Build history of the part. All positions in model axes, mm. Round coordinates to 2 decimals unless told otherwise and drop trailing zeros. Write each loop counter-clockwise with the first axis right and the second up, starting at its lowest first coordinate (ties: lowest second). Pieces come first, ordered by that corner, then holes. Notation, with made-up numbers: (87, 80.25) -> (123, 80.25) arc R13 cw to (123, 87.25) -> close; hole circle Ø6 at (89, 57). An arc over 180 degrees is marked (long way). One line per question, with ' | ' between items.
Autodesk Inventor part; units mm, degrees
ref_plane "YZ Plane" through (0, 0, 0) normal (1, 0, 0) x (0, 1, 0)
ref_plane "XZ Plane" through (0, 0, 0) normal (0, 1, 0) x (-1, 0, 0)
ref_plane "XY Plane" through (0, 0, 0) normal (0, 0, 1) x (1, 0, 0)
sketch "Sketch1" plane through (0, 0, 0) normal (0, 1, 0) x (-1, 0, 0)
  line L0 (0, 0) -> (4.2574, -0.7507)
  line L1 (4.8854, -1.4991) -> (4.8854, -10.87)
  line L2 (0, 0) -> (-0.1146, -0.65)
  line L3 (-0.1146, -0.65) -> (4.1428, -1.4007)
  line L4 (4.2254, -1.4991) -> (4.2254, -10.87)
  line L5 (4.8854, -7.3684) -> (4.2254, -7.3684) construction
  arc A0 (4.8854, -1.4991) -> (4.2574, -0.7507) centre (4.1254, -1.4991) ccw
  arc A1 (4.2254, -1.4991) -> (4.1428, -1.4007) centre (4.1254, -1.4991) ccw
  line L6 (0, 0) -> (9.7928, 0) construction
  arc A2 (4.2254, -10.87) -> (7.5579, -14.4878) centre (7.8554, -10.87) ccw
  arc A3 (4.8854, -10.87) -> (7.1313, -13.7504) centre (7.8554, -10.87) ccw
  arc A4 (7.1313, -13.7504) -> (5.1401, -11.0799) centre (5.0441, -13.2291) ccw
  line L7 (7.1313, -13.7504) -> (6.9714, -14.3907) construction
  line L8 (7.1313, -13.7504) -> (7.7714, -13.9113) construction
  line L9 (5.1401, -11.0799) -> (5.1689, -10.4206)
  arc A5 (7.5579, -14.4878) -> (5.1689, -10.4206) centre (5.0441, -13.2291) ccw
  line L10 (7.8554, -14.5) -> (1.0376, -14.5) construction
  line L11 (7.8554, -14.5) -> (7.8554, -9.8671) construction
  dimension "d0" = 0.66
  dimension "d2" = 10
  dimension "d3" = 0.1
  dimension "d4" = 14.5
  dimension "d5" = 5
  dimension "d6" = 3.63
  dimension "d8" = 2.5
  dimension "d9" = 4.0794
extrude "Extrusion1" add sketch "Sketch1" along normal blind 4.7
fillet "Fillet1" radius 0.5 1 edges at (-7.5579, 2.35, -14.4878)
sketch "Sketch2" plane through (0, 0, 0) normal (-0.1736, 0, 0.9848) x (0.9848, 0, 0.1736)
  line L0 (-4.323, 4.7) -> (0, 4.7)
  line L1 (0, 0) -> (-4.323, 0)
  line L2 (-1, 4.7) -> (-0.25, 4.7)
  line L3 (-0.25, 4.7) -> (-0.25, 6.2)
  line L4 (-0.25, 6.2) -> (-1, 6.2)
  line L5 (-1, 6.2) -> (-1, 4.7)
  line L6 (-1, 0) -> (-0.25, 0)
  line L7 (-0.25, 0) -> (-0.25, -1.5)
  line L8 (-0.25, -1.5) -> (-1, -1.5)
  line L9 (-1, -1.5) -> (-1, 0)
  line L10 (0, 0) -> (0, 4.7)
  dimension "d13" = 1.5
  dimension "d14" = 0.75
  dimension "d15" = 0.25
extrude "Extrusion2" add sketch "Sketch2" against normal up to surface (0.66 mm away)
properties part number "Lever" material "Stainless Steel"
(1) Mould opens along X. For faces 1 (the flat face through (-4.7, 0, -7.7)), 2 (the cylindrical face through (-6.75, 2.32, -11.92)), 3 (the cylindrical face through (-5.53, 2.32, -12.72)), 4 (the flat face through (-1.98, 2.32, -1.02)) say: pulls with the +X half, pulls with the -X half, needs draft (parallel to the pull), parting line crosses it, or undercut.
Calculated:
face 1: needs draft | face 2: undercut | face 3: undercut | face 4: pulls with the +X half
(2) Slice it at B-B (y = -1). Write the cut outline in (x, z).
Calculated:
outline: (-0.98, -0.17) -> (-0.87, -0.82) -> (-0.13, -0.69) -> (-0.25, -0.04) -> close
(3) Drop flat-ended pins along their axis: pin 1 (4 mm diameter, centred on x = -5.5, z = -4, fed in from +Y); pin 2 (2.5 mm diameter, centred on y = 1.5, z = -5, fed in from +X); pin 3 (1 mm diameter, centred on x = -5.5, y = 4.5, fed in from -Z); pin 4 (1 mm diameter, centred on x = -6.5, z = -8, fed in from -Y). Give the stop position or say it passes through.
Calculated:
pin 1: y = 4.7 | pin 2: x = -4.23 | pin 3: z = -13.99 | pin 4: through
(4) Wall check: line 1 (X direction, y = 0.25, z = -5); line 2 (X direction, y = 4.5, z = -13); line 3 (Y direction, x = -2.5, z = -1). Give the ranges that are in metal, low to high. Write a range as from..to.
Calculated:
line 1: -4.89..-4.23 | line 2: -7.85..-7.18, -5.79..-4.92 | line 3: 0..4.7
(5) Slice it at A-A (x = -6.75). Write the cut outline in (y, z), then the cut area to 3 significant figures.
Calculated:
outline: (0, -14.33) -> (4.7, -14.33) -> (4.7, -13.63) -> (0, -13.63) -> close; (0, -11.92) -> (4.7, -11.92) -> (4.7, -10.99) -> (0, -10.99) -> close | area: 7.64 mm2
(6) Slice it at C-C (z = -8.75). Write the cut outline in (x, y).
Calculated:
outline: (-4.89, 0) -> (-4.23, 0) -> (-4.23, 4.7) -> (-4.89, 4.7) -> close
